Part model, mm, in its own coordinate system. Coordinates: 2 decimals unless noted, no trailing zeros. Loops run counter-clockwise (first coordinate to the right, second up) from the corner with the lowest first, then second, coordinate; pieces in that order, holes last. Notation, with made-up numbers: M 36.25,48 L 43.25,48 A12 cw 43.25,65 Z; hole C 63.5,-4.5 d2. An arc over 180 degrees is marked long. Answer as a JSON object with one key per item and string values. Group by question number.
1. Saw through at B-B on z = 8. Write the cut outline in (x, y), then the cut area to 3 significant figures.
2. Saw through at A-A on z = 56. Write the cut outline in (x, y).
3. Drill centre lines: L1, parallel to X at y = 0, z = 3; L2, parallel to Y at x = 0, z = 2.75. Where is each one in solid material? Low to high.
4. Mould opens along X. For faces 1 (the face through (0, 0, 0)), 2 (the face through (-4.094, 7.871, 32.045)), 3 (the face through (-0.217, -11.524, 2.465)) say: released by +X, released by -X, zero draft, split by the parting line, or undercut.
5. Drop flat-ended pins along their axis: pin 1 Ø1.2 at (x, y) = (0, -12.5) entering from -Z; pin 2 Ø6 at (y, z) = (-2, 41.5) entering from +X; pin 3 Ø10 at (y, z) = (2.5, 8.5) entering from +X. Give the stop position or say it passes through.
from build123d import *

# Parameters (mm, degrees)
F2_R     = 1
F3_DEPTH = 5


with BuildPart() as f1:
    # F0 (on Front) → F1 (revolve)
    with BuildSketch(Plane.XZ):
        Polygon((-17.5, 0), (0, 0), (0, 65), align=None)
    revolve(axis=Axis((0, 0, 32.5), (0, 0, 1)))

    # F2 (on face) → F3 (cut)
    with BuildSketch(Plane(origin=(0, 0, 0), x_dir=(1, 0, 0), z_dir=(0, 0, -1))):
        with Locations((0, -12.5)):
            Circle(F2_R)
        with Locations((-12.5, 0)):
            Circle(F2_R)
        with Locations((0, 12.5)):
            Circle(F2_R)
        with Locations((12.5, 0)):
            Circle(F2_R)
    extrude(amount=-F3_DEPTH, mode=Mode.SUBTRACT)


solid = f1.part
Outcome:
{
 "1": {"outline": "C 0,0 d30.69", "area": "740 mm²"},
 "2": {"outline": "C 0,0 d4.85"},
 "3": {"L1": "x = -16.69 to -13.5, -11.5 to 11.5, 13.5 to 16.69", "L2": "y = -16.76 to -13.5, -11.5 to 11.5, 13.5 to 16.76"},
 "4": {"face 1": "zero draft", "face 2": "split by the parting line", "face 3": "undercut"},
 "5": {"pin 1": "stops at z = 5", "pin 2": "stops at x = 7.02", "pin 3": "stops at x = 16.47"}
}
